Check sheet for the drawn part. Datum: minimum x, y, z corner. Units: mm. A direction names the side the tool comes from. Coordinates: 2 decimals unless noted, no trailing zeros. Loops run counter-clockwise (first coordinate to the right, second up) from the corner with the lowest first, then second, coordinate; pieces in that order, holes last. Notation, with made-up numbers: (71.25, -18.75) - (120.25, -18.75) arc R33 ccw to (120.25, 9.25) - close; hole circle Ø9 at (-13.5, -35). An arc over 180 degrees is marked (long way). Answer as a JSON object with one key per item and string values. Group by question number.
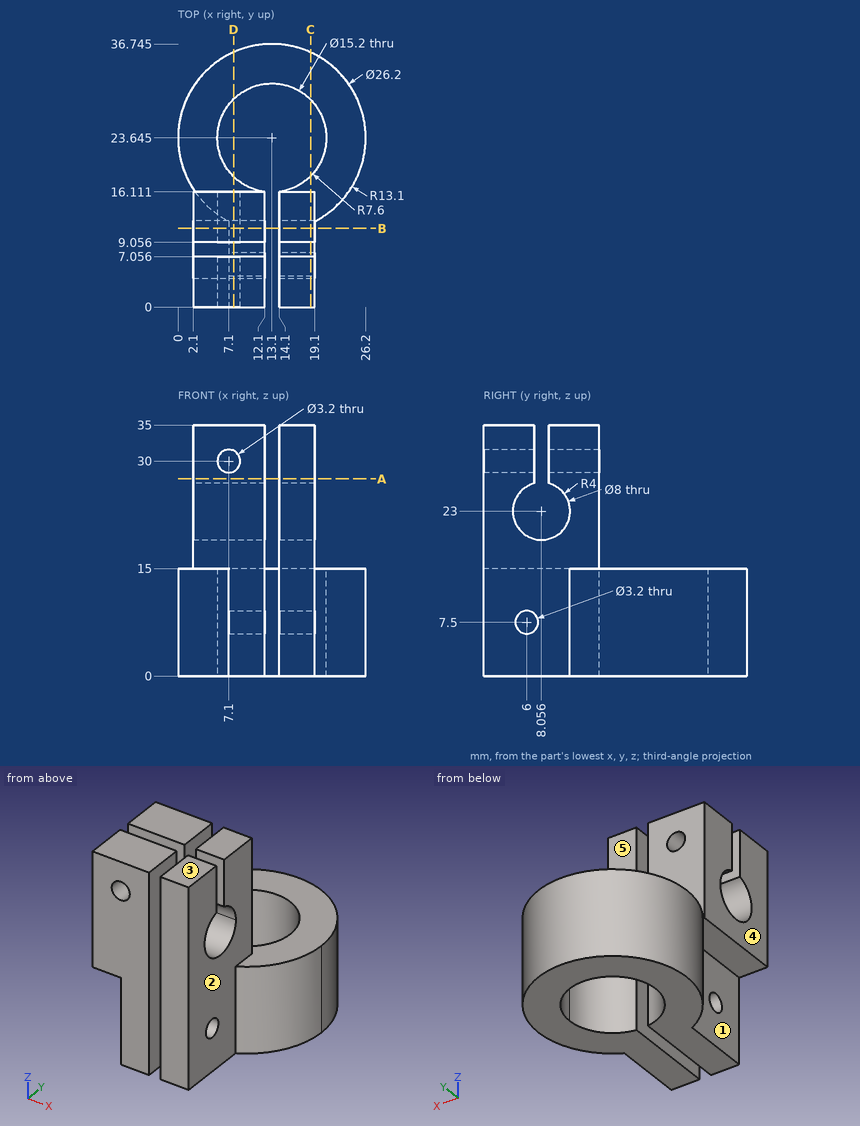
1. Material ranges on line 1 (X direction, y = 3, z = 22.5); line 2 (Y direction, x = 9.5, z = 30.5) (1 decimal); line 3 (X direction, y = 14, z = 12.5) (1 decimal), recorded low to high.
2. Access from +Z, -Z, +X, -X, +Y, -Y to the whole of each face (thin tool, end or side, straight path). Record for the marked faces 1, 2, 3, 4 and 5.
3. Sectioned sample at D-D on x = 7.75. Record the cut outline in (y, z) (1 decimal), plus the area to 3 significant figures.
4. Sectioned sample at C-C on x = 18.5. Record the cut outline in (y, z) (1 decimal), plus the area to 3 significant figures.
5. Sectioned sample at A-A on z = 27.5. Record the cut outline in (x, y) (1 decimal), plus the area to 3 significant figures.
6. Sectioned sample at B-B on y = 11. Record the cut outline in (x, z).
7. Gauge pin test, flat ends, axial feed: pin 1 (7.5 mm diameter, centred on x = 14, y = 28.5, fed in from +Z); pin 2 (13 mm diameter, centred on y = 8.06, z = 23, fed in from +X); pin 3 (4 mm diameter, centred on x = 2.5, y = 6.5, fed in from -Z). Record the tip position at first contact, or that the pin passes through.
Answers follow:
{
 "1": {"line 1": "x = 2.1 to 12.1, 14.1 to 19.1", "line 2": "y = 0 to 7.1, 9.1 to 16.1", "line 3": "x = 4.2 to 12.1, 14.1 to 22"},
 "2": {"face 1": "-Z, -X, -Y", "face 2": "+Z, +X, -Y", "face 3": "+Z, +X, -X, +Y, -Y", "face 4": "+Z, -Z, -X, +Y, -Y", "face 5": "+Z, +X, -X, +Y"},
 "3": {"outline": "(0, 0) - (18.2, 0) - (18.2, 15) - (16.1, 15) - (16.1, 28.5) - (9.1, 28.5) - (9.1, 26.9) arc R4 cw (long way) to (7.1, 26.9) - (7.1, 28.5) - (0, 28.5) - close; (0, 31.5) - (7.1, 31.5) - (7.1, 35) - (0, 35) - close; (9.1, 31.5) - (16.1, 31.5) - (16.1, 35) - (9.1, 35) - close; (29, 0) - (35.6, 0) - (35.6, 15) - (29, 15) - close; hole circle Ø3.2 at (6, 7.5)", "area": "579 mm^2"},
 "4": {"outline": "(0, 0) - (18.3, 0) - (18.3, 15) - (16.1, 15) - (16.1, 35) - (9.1, 35) - (9.1, 26.9) arc R4 cw (long way) to (7.1, 26.9) - (7.1, 35) - (0, 35) - close; (29, 0) - (35.6, 0) - (35.6, 15) - (29, 15) - close; hole circle Ø3.2 at (6, 7.5)", "area": "621 mm^2"},
 "5": {"outline": "(2.1, 0) - (12.1, 0) - (12.1, 7.1) - (2.1, 7.1) - close; (2.1, 9.1) - (12.1, 9.1) - (12.1, 16.1) - (2.1, 16.1) - close; (14.1, 0) - (19.1, 0) - (19.1, 7.1) - (14.1, 7.1) - close; (14.1, 9.1) - (19.1, 9.1) - (19.1, 16.1) - (14.1, 16.1) - close", "area": "212 mm^2"},
 "6": {"outline": "(2.1, 15) - (7.1, 15) - (7.1, 0) - (12.1, 0) - (12.1, 20.29) - (2.1, 20.29) - close; (2.1, 25.71) - (12.1, 25.71) - (12.1, 35) - (2.1, 35) - close; (14.1, 0) - (19.1, 0) - (19.1, 20.29) - (14.1, 20.29) - close; (14.1, 25.71) - (19.1, 25.71) - (19.1, 35) - (14.1, 35) - close; hole circle Ø3.2 at (7.1, 30)"},
 "7": {"pin 1": "stops at z = 15", "pin 2": "stops at x = 19.1", "pin 3": "stops at z = 15"}
}
